The listing builds one solid part. Answer for the finished solid, in the listing's coordinates (mm). A direction names the side the tool comes from. Give positions to 0.01 mm unless a question says otherwise; leave off trailing zeros. Write each loop counter-clockwise with the first axis right and the second up, starting at its lowest first coordinate (ties: lowest second). Pieces come first, ordered by that corner, then holes. Notation, with made-up numbers: (37.5, 11.25) -> (59.5, 11.25) arc R16 ccw to (59.5, 15.25) -> close; hole circle Ø10 at (73, 15.5). An arc over 180 degrees is marked (long way). Put each result on its own line as item: value. Start each with the question number.
1) A cutting plane is placed at D-D (y = -11.5). Write down the section's boundary in (x, z).
2) A cutting plane is placed at B-B (x = 0). Write down the section's boundary in (y, z), then the cut area to 3 significant figures.
3) Find the intervals of material crossed by line 1 along Z through (x, y) = (40, -25.75); line 2 along Z through (x, y) = (19, -28); line 3 along Y through (x, z) = (-2, 16), in increasing order. Write a range as from..to.
4) A cutting plane is placed at C-C (z = -5). Write down the section's boundary in (x, y), then the cut area to 3 significant figures.
5) For faces 4 (the cylindrical face through (20.18, -30.07, -15.08)), 5 (the flat face through (30, -31, 5)), 6 (the flat face through (30, -13, 5)), 7 (the cylindrical face through (2.285, 3.584, 14.93)), determine the directions among +Z, -Z, +X, -X, +Y, -Y from which every point of the face is accessible in a straight line to the end or side of a thin tool.
6) A cutting plane is placed at A-A (z = -14). Write down the section's boundary in (x, y), then the cut area to 3 significant figures.
7) For a pull along X with two mould halves and no side action, classify faces 1 (the flat face through (40, -27.4, 5)), 2 (the cylindrical face through (0.66, 24.993, 5.056)), 3 (the cylindrical face through (41.65, -23.75, -5.07)) as released by +X, released by -X, zero draft, split by the parting line, or undercut.
8) Flat-ended cylindrical pins translate along their axes: pin 1 Ø4 at (x, y) = (19.5, 13) entering from -Z; pin 2 Ø3 at (y, z) = (7, 17.5) entering from +X; pin 3 Ø2 at (x, z) = (38.5, 19.5) entering from +Y; pin 4 Ø4 at (y, z) = (-12.5, 5.5) entering from +X. Find the tip coordinate at first contact, or state that the pin passes through.
from build123d import *

# Parameters (mm, degrees)
SKETCH_1_W          = 60
SKETCH_1_H          = 50
EXTRUDE_1_DEPTH     = 10
SKETCH_8_W          = 80
SKETCH_8_H          = 60
EXTRUDE_2_DEPTH     = 10
SKETCH_9_R          = 4.75
SKETCH_9_R_2        = 4.25
EXTRUDE_3_DEPTH     = 10
SKETCH_11_W         = 20
SKETCH_11_H         = 7.6
CUT_EXTRUDE_1_DEPTH = 21
SKETCH_12_W         = 20
SKETCH_12_H         = 5
EXTRUDE_4_DEPTH     = 30
HOLE_WIZARD_4_D     = 3.3
EXTRUDE_START       = -60
EXTRUDE_5_DEPTH     = 60
FILLET_1_RADIUS     = 30
FILLET_1_LENGTH     = 10
CHAMFER_1_SIZE      = 1
HOLE_WIZARD_5_D     = 3.2


with BuildPart() as part:
    # 草图1 → 凸台-拉伸1 (new body)
    with BuildSketch(Plane.XY):
        Rectangle(SKETCH_1_W, SKETCH_1_H)
    extrude(amount=EXTRUDE_1_DEPTH)

    # 草图3 → 孔1 (revolve, cut)
    with BuildSketch(Plane(origin=(0, 0, 10), x_dir=(0, -1, 0), z_dir=(1, 0, 0))):
        Polygon((0, 0), (0, 10), (4, 10), (4, 0.603553391), (4.25, 0), align=None)
    revolve(axis=Axis((0, 0, 16.445314094), (0, 0, -1)), mode=Mode.SUBTRACT)

    # 草图8 → 凸台-拉伸2 (add)
    with BuildSketch(Plane.XZ.offset(25)):
        with Locations((10, 5)):
            Rectangle(SKETCH_8_W, SKETCH_8_H)
    extrude(amount=EXTRUDE_2_DEPTH)

    # 草图9 → 凸台-拉伸3 (add)
    with BuildSketch(Plane.XY.offset(10)):
        with Locations(Location((0, 0, 0), (0, 0, 180))):
            Circle(SKETCH_9_R)
        Circle(SKETCH_9_R_2, mode=Mode.SUBTRACT)
    extrude(amount=EXTRUDE_3_DEPTH)

    # 草图11 → 切除-拉伸1 (cut, symmetric)
    with BuildSketch(Plane.XY.offset(5)):
        with Locations((40, -31.2)):
            Rectangle(SKETCH_11_W, SKETCH_11_H)
    extrude(amount=CUT_EXTRUDE_1_DEPTH, both=True, mode=Mode.SUBTRACT)

    # 草图12 → 凸台-拉伸4 (add, symmetric)
    with BuildSketch(Plane.XY.offset(5)):
        with Locations((40, -22.5)):
            Rectangle(SKETCH_12_W, SKETCH_12_H)
    extrude(amount=EXTRUDE_4_DEPTH, both=True)

    # 孔4 (through all)
    with Locations(Plane(origin=(0, -20, 0), x_dir=(1, 0, 0), z_dir=(0, 1, 0))):
        with Locations((40, -15), (40, 5)):
            Hole(HOLE_WIZARD_4_D / 2)

    # 草图15 → 凸台-拉伸5 (add)
    with BuildSketch(Plane.XY.offset(35).offset(EXTRUDE_START)):
        Polygon((30, -20), (22.5, -25), (30, -25), align=None)
    extrude(amount=EXTRUDE_5_DEPTH)

    # 圆角1: full round fillet: the end face becomes a half cylinder, R = half its width
    fillet_1_face = Plane((0, 25, 5), x_dir=(0, 0, 1), z_dir=(0, 1, 0))  # on the end face: x along it, z out of the body
    fillet_1_slab = fillet_1_face.offset(-FILLET_1_RADIUS / 2) * Box(FILLET_1_LENGTH, 2 * FILLET_1_RADIUS, FILLET_1_RADIUS, mode=Mode.PRIVATE)  # the body's end, R deep
    fillet_1_round = Plane((0, -5, 5), x_dir=(0, 1, 0), z_dir=(0, 0, 1)) * Cylinder(FILLET_1_RADIUS, FILLET_1_LENGTH, mode=Mode.PRIVATE)  # its axis R under the face
    add(fillet_1_slab - fillet_1_round, mode=Mode.SUBTRACT)

    # 倒角1
    chamfer_1_edges = [part.edges().sort_by_distance(p)[0] for p in [
        (26.25, -22.5, -25),
        (26.25, -22.5, 35),
        (-30, -15, 0),
        (-30, -15, 10),
        (0, 25, 10),
        (0, 25, 0),
        (-30, -25, 22.5),
        (-30, -25, -12.5),
        (-30, -30, 35),
        (-3.75, -25, -25),
        (-30, -30, -25),
        (30, -12.5, 0),
        (30, -12.5, 10),
        (-3.75, -25, 35),
    ]]
    chamfer(chamfer_1_edges, length=CHAMFER_1_SIZE)

    # 孔5 (through all)
    with Locations(Plane(origin=(0, -25, 0), x_dir=(1, 0, 0), z_dir=(0, 1, 0))):
        with Locations((-19, 14), (19, 14), (19, -24), (-19, -24)):
            Hole(HOLE_WIZARD_5_D / 2)


solid = part.part
Reply:
1. outline: (-30, 1) -> (-29, 0) -> (29, 0) -> (30, 1) -> (30, 9) -> (29, 10) -> (-29, 10) -> (-30, 9) -> close
2. outline: (-35, -25) -> (-26, -25) -> (-25, -24) -> (-25, 0) -> (-4, 0) -> (-4, 9.4) -> (-4.25, 10) -> (-4.25, 20) -> (-4.75, 20) -> (-4.75, 10) -> (-25, 10) -> (-25, 34) -> (-26, 35) -> (-35, 35) -> close; (4, 0) -> (24, 0) -> (25, 1) -> (25, 9) -> (24, 10) -> (4.75, 10) -> (4.75, 20) -> (4.25, 20) -> (4.25, 10) -> (4, 9.4) -> close
2. area: 1,030 mm2
3. line 1: z = -25..-6.65, -3.35..13.35, 16.65..35
3. line 2: z = -25..-15.6, -12.4..22.4, 25.6..35
3. line 3: y = -35..-25, -4.31..-3.75, 3.75..4.31
4. outline: (-30, -35) -> (30, -35) -> (30, -27.4) -> (38.35, -27.4) -> (38.35, -20) -> (30, -20) -> (22.5, -25) -> (-29, -25) -> (-30, -26) -> close; (41.65, -27.4) -> (50, -27.4) -> (50, -20) -> (41.65, -20) -> close
4. area: 742 mm2
5. face 4: +Y, -Y
5. face 5: +X, -Y
5. face 6: +Z, -Z, +X, +Y
5. face 7: +Z
6. outline: (-30, -35) -> (-20.6, -35) -> (-20.6, -25) -> (-29, -25) -> (-30, -26) -> close; (-17.4, -35) -> (17.4, -35) -> (17.4, -25) -> (-17.4, -25) -> close; (20.6, -35) -> (30, -35) -> (30, -27.4) -> (50, -27.4) -> (50, -20) -> (30, -20) -> (22.5, -25) -> (20.6, -25) -> close
6. area: 702 mm2
7. face 1: zero draft
7. face 2: split by the parting line
7. face 3: undercut
8. pin 1: stops at z = 0
8. pin 2: passes through
8. pin 3: stops at y = -20
8. pin 4: stops at x = 30
